Design review of the part built by this model. Coordinates are the model's own, in mm. Face numbers are marked on the shaded views. A direction names the side the tool comes from. Give positions to 0.01 mm unless a question says otherwise; leave off trailing zeros. Write each loop counter-clockwise with the first axis right and the second up, starting at its lowest first coordinate (ties: lowest second). Pieces come first, ordered by that corner, then holes.
```python
from build123d import *

# Parameters (mm, degrees)
SKETCH2_W           = 3.6
SKETCH2_H           = 3.6
BOSS_EXTRUDE1_DEPTH = 40
SKETCH3_R           = 10
BOSS_EXTRUDE2_DEPTH = 4
SKETCH5_W           = 10
SKETCH5_H           = 1.075357982
BOSS_EXTRUDE3_DEPTH = 15
FILLET3_RADIUS      = 5
FILLET3_LENGTH      = 1.075357982
FILLET4_RADIUS      = 5
FILLET4_LENGTH      = 1.075357982
CUT_EXTRUDE1_REACH  = 64.683
SKETCH6_R           = 1


with BuildPart() as part:
    # Sketch2 → Boss-Extrude1 (new body)
    with BuildSketch(Plane(origin=(0, 0, 0), x_dir=(1, 0, 0), z_dir=(0, 1, 0))):
        Rectangle(SKETCH2_W, SKETCH2_H)
    extrude(amount=BOSS_EXTRUDE1_DEPTH)

    # Sketch3 → Boss-Extrude2 (add)
    with BuildSketch(Plane(origin=(0, 40, 0), x_dir=(1, 0, 0), z_dir=(0, 1, 0))):
        with Locations(Location((0, 0, 0), (0, 0, 270))):
            Circle(SKETCH3_R)
    extrude(amount=BOSS_EXTRUDE2_DEPTH)

    # Sketch5 → Boss-Extrude3 (add)
    with BuildSketch(Plane(origin=(0, 44, 0), x_dir=(1, 0, 0), z_dir=(0, 1, 0))):
        with Locations((0, 8.122575047)):
            Rectangle(SKETCH5_W, SKETCH5_H)
        with Locations((0, -8.122575047)):
            Rectangle(SKETCH5_W, SKETCH5_H)
    extrude(amount=BOSS_EXTRUDE3_DEPTH)

    # Fillet3: full round fillet: the end face becomes a half cylinder, R = half its width
    fillet3_face = Plane((0, 59, 8.122575047), x_dir=(0, 0, -1), z_dir=(0, 1, 0))  # on the end face: x along it, z out of the body
    fillet3_slab = fillet3_face.offset(-FILLET3_RADIUS / 2) * Box(FILLET3_LENGTH, 2 * FILLET3_RADIUS, FILLET3_RADIUS, mode=Mode.PRIVATE)  # the body's end, R deep
    fillet3_round = Plane((0, 54, 8.122575047), x_dir=(0, 1, 0), z_dir=(0, 0, -1)) * Cylinder(FILLET3_RADIUS, FILLET3_LENGTH, mode=Mode.PRIVATE)  # its axis R under the face
    add(fillet3_slab - fillet3_round, mode=Mode.SUBTRACT)

    # Fillet4: full round fillet: the end face becomes a half cylinder, R = half its width
    fillet4_face = Plane((0, 59, -8.122575047), x_dir=(0, 0, 1), z_dir=(0, 1, 0))  # on the end face: x along it, z out of the body
    fillet4_slab = fillet4_face.offset(-FILLET4_RADIUS / 2) * Box(FILLET4_LENGTH, 2 * FILLET4_RADIUS, FILLET4_RADIUS, mode=Mode.PRIVATE)  # the body's end, R deep
    fillet4_round = Plane((0, 54, -8.122575047), x_dir=(0, 1, 0), z_dir=(0, 0, 1)) * Cylinder(FILLET4_RADIUS, FILLET4_LENGTH, mode=Mode.PRIVATE)  # its axis R under the face
    add(fillet4_slab - fillet4_round, mode=Mode.SUBTRACT)

    # Cut-Extrude1: up to this face of the body (flat: up to its plane)
    cut_extrude1_end = Plane(part.part.faces().sort_by_distance((0, 51.008207501, -8.660254038))[0])
    # Sketch6 → Cut-Extrude1 (cut, up to the picked face)
    with BuildSketch(Plane.XY.offset(8.660254038), mode=Mode.PRIVATE) as cut_extrude1_sk1:
        with Locations((0, 54)):
            Circle(SKETCH6_R)
    cut_extrude1_tool1 = split(extrude(cut_extrude1_sk1.sketch, amount=-CUT_EXTRUDE1_REACH, mode=Mode.PRIVATE), bisect_by=cut_extrude1_end, keep=Keep.BOTH, mode=Mode.PRIVATE)
    add(cut_extrude1_tool1.solids().sort_by(Axis((0, 54, 8.660254), (0, 0, -1)))[0], mode=Mode.SUBTRACT)


solid = part.part
```
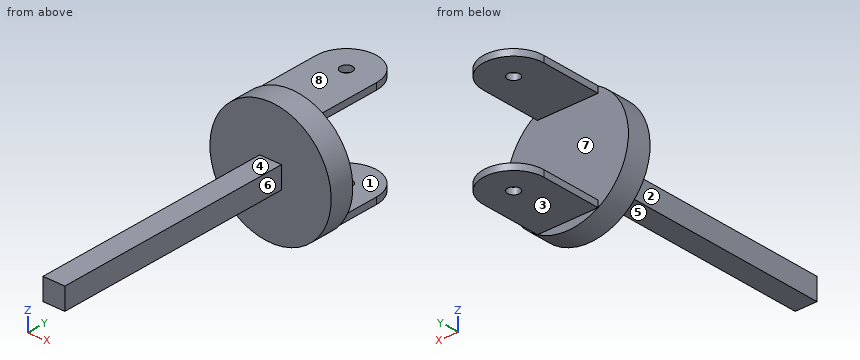
(1) To check wall thickness, follow L1, parallel to Z at x = 1, y = 52; L2, parallel to Y at x = 0, z = 8.05; L3, parallel to Y at x = 8.5, z = 1. State the ranges of each line that lie inside material, in increasing order.
Resolved:
L1: z = -8.66 to -7.58, 7.58 to 8.66
L2: y = 40 to 53, 55 to 59
L3: y = 40 to 44
(2) Consider section D-D, the plane x = 3.75. Give the boundary of the cut face in (y, z).
Resolved:
outline: (40, -9.27) - (44, -9.27) - (44, -8.66) - (57.31, -8.66) - (57.31, -7.58) - (44, -7.58) - (44, 7.58) - (57.31, 7.58) - (57.31, 8.66) - (44, 8.66) - (44, 9.27) - (40, 9.27) - close
(3) Clearance check with flat-ended pins moving along their axes: P1, Ø1.5, axis at y = 24, z = 1, coming from the +X side; P2, Ø6, axis at y = 49.5, z = 5, coming from the +X side; P3, Ø5, axis at x = -5.5, y = 42.5, coming from the -Z side. State where each tip first meets the part, or that it passes through.
Resolved:
P1: stops at x = 1.8
P2: stops at x = 5
P3: stops at z = -9.54
(4) Consider section A-A, the plane x = 0. Give the boundary of the cut face in (y, z).
Resolved:
outline: (0, -1.8) - (40, -1.8) - (40, -10) - (44, -10) - (44, -8.66) - (53, -8.66) - (53, -7.58) - (44, -7.58) - (44, 7.58) - (53, 7.58) - (53, 8.66) - (44, 8.66) - (44, 10) - (40, 10) - (40, 1.8) - (0, 1.8) - close; (55, -8.66) - (59, -8.66) - (59, -7.58) - (55, -7.58) - close; (55, 7.58) - (59, 7.58) - (59, 8.66) - (55, 8.66) - close
(5) Tool access review of the marked faces 1, 2, 3, 4 and 5: name each direction out of +Z, -Z, +X, -X, +Y, -Y from which nothing blocks a thin tool from reaching the whole face with its end or side.
Resolved:
face 1: +X, -X, +Y
face 2: +Z, -Z, -X, -Y
face 3: -Z, +X, -X, +Y
face 4: +Z, +X, -X, -Y
face 5: -Z, +X, -X, -Y
(6) Consider section C-C, the plane z = 0. Give the boundary of the cut face in (x, y), then the cut area to 3 significant figures.
Resolved:
outline: (-10, 40) - (-1.8, 40) - (-1.8, 0) - (1.8, 0) - (1.8, 40) - (10, 40) - (10, 44) - (-10, 44) - close
area: 224 mm2
(7) Consider section B-B, the plane y = 47.5. Give the boundary of the cut face in (x, z).
Resolved:
outline: (-5, -8.66) - (5, -8.66) - (5, -7.58) - (-5, -7.58) - close; (-5, 7.58) - (5, 7.58) - (5, 8.66) - (-5, 8.66) - close
(8) Mouldability with a two-part tool opening along Z and no side actions: class the marked faces 6, 7 and 8 as pulls with the +Z half, pulls with the -Z half, needs draft (parallel to the pull), parting line crosses it, or undercut.
Resolved:
face 6: needs draft
face 7: undercut
face 8: pulls with the +Z half
